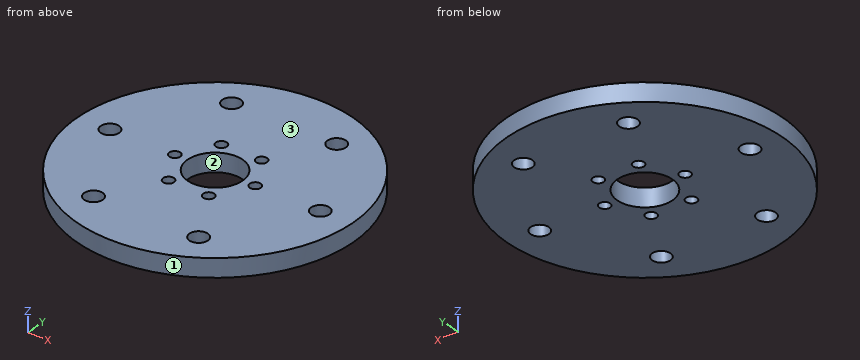
Autodesk Inventor part; units mm, degrees
ref_plane "YZ Plane" through (0, 0, 0) normal (1, 0, 0) x (0, 1, 0)
ref_plane "XZ Plane" through (0, 0, 0) normal (0, 1, 0) x (-1, 0, 0)
ref_plane "XY Plane" through (0, 0, 0) normal (0, 0, 1) x (1, 0, 0)
sketch "Sketch1" plane through (0, 0, 0) normal (0, 0, 1) x (1, 0, 0)
  circle A0 centre (0, 0) radius 37.5
  circle A1 centre (0, 0) radius 7.5
  circle A2 centre (28.75, 0) radius 2.5
  circle A3 centre (11, 0) radius 1.5
  circle A4 centre (14.375, 24.8982) radius 2.5
  circle A5 centre (5.5, 9.5263) radius 1.5
  circle A6 centre (-14.375, 24.8982) radius 2.5
  circle A7 centre (-5.5, 9.5263) radius 1.5
  circle A8 centre (-28.75, 0) radius 2.5
  circle A9 centre (-11, 0) radius 1.5
  circle A10 centre (-14.375, -24.8982) radius 2.5
  circle A11 centre (-5.5, -9.5263) radius 1.5
  circle A12 centre (14.375, -24.8982) radius 2.5
  circle A13 centre (5.5, -9.5263) radius 1.5
  dimension "d0" = 75
  dimension "d1" = 15
  dimension "d2" = 5
  dimension "d3" = 3
  dimension "d4" = 28.75
  dimension "d5" = 11
  dimension "d8" = 360
extrude "Extrusion1" add sketch "Sketch1" along normal blind 5
properties part number "TA04" material "ABS Plastic"
The listing builds one solid part. Answer for the finished solid, in the listing's coordinates (mm). Face numbers are marked on the shaded views. Coordinates: 2 decimals unless noted, no trailing zeros. Write each loop counter-clockwise with the first axis right and the second up, starting at its lowest first coordinate (ties: lowest second). Pieces come first, ordered by that corner, then holes. Notation, with made-up numbers: (52, 40.5) - (60, 40.5) arc R24 ccw to (60, 59.5) - close; hole circle Ø3 at (-29.5, 13.25). An arc over 180 degrees is marked (long way). Return JSON: item names as keys, results as strings. Group by question number.
Q1. The part is cut by section C-C on x = -15.5. Write down the section's boundary in (y, z), and give its area (3 significant figures).
Q2. For a pull along Y with two mould halves and no side action, classify the marked faces 1, 2 and 3 as +Y half, -Y half, draft (parallel to the pull), parting line (faces both ways), or undercut.
Q3. Flat-ended cylindrical pins translate along their axes: pin 1 Ø3 at (y, z) = (-17, 4) entering from +X; pin 2 Ø1 at (y, z) = (12, 0.5) entering from +X. Find the tip coordinate at first contact, or state that the pin passes through.
Q4. Find the intervals of material crossed by line 1 along Y through (x, z) = (15.5, 2.6); line 2 along X through (y, z) = (-26, 3.75); line 3 along Y through (x, z) = (5.5, 2.35), in increasing order. Write a range as [from, to].
Q5. The part is cut by section D-D on x = 11. Write down the section's boundary in (y, z).
Q6. The part is cut by section A-A on x = 0. Write down the section's boundary in (y, z).
Q7. The part is cut by section B-B on z = 1.9. State how many separate pieces and enclosed holes the cut face has, and give its area (3 significant figures).
Evaluation:
{
 "1": {"outline": "(-34.15, 0) - (-27.13, 0) - (-27.13, 5) - (-34.15, 5) - close; (-22.67, 0) - (22.67, 0) - (22.67, 5) - (-22.67, 5) - close; (27.13, 0) - (34.15, 0) - (34.15, 5) - (27.13, 5) - close", "area": "297 mm2"},
 "2": {"face 1": "parting line", "face 2": "undercut", "face 3": "draft"},
 "3": {"pin 1": "stops at x = 34.15", "pin 2": "stops at x = 35.69"},
 "4": {"line 1": "y = [-34.15, -27.13], [-22.67, 22.67], [27.13, 34.15]", "line 2": "x = [-27.02, -16.62], [-12.13, 12.13], [16.62, 27.02]", "line 3": "y = [-37.09, -11.03], [-8.03, -5.1], [5.1, 8.03], [11.03, 37.09]"},
 "5": {"outline": "(-35.85, 0) - (-1.5, 0) - (-1.5, 5) - (-35.85, 5) - close; (1.5, 0) - (35.85, 0) - (35.85, 5) - (1.5, 5) - close"},
 "6": {"outline": "(-37.5, 0) - (-7.5, 0) - (-7.5, 5) - (-37.5, 5) - close; (7.5, 0) - (37.5, 0) - (37.5, 5) - (7.5, 5) - close"},
 "7": {"separate pieces": "1", "enclosed holes": "13", "area": "4,080 mm2"}
}
